Geometry check sheet. Reference: drawing and pictorial views, mm from the part's lowest x, y, z. A direction names the side the tool comes from. Give positions to 0.01 mm unless a question says otherwise; leave off trailing zeros. Order: outer loops, then holes, each group sorted by start corner. A loop starts at its lowest first (then second) coordinate and runs counter-clockwise, first axis right, second up.
Item 1: Release check for a two-part mould opening along X. For the marked faces 3, 4 and 5 record: released by +X, released by -X, zero draft, split by the parting line, or undercut.
Item 2: Sectioned sample at C-C on x = 32.5. Record the boundary of the cut face in (y, z).
Item 3: Gauge pin test, flat ends, axial feed: P1, Ø1, axis at x = 28, z = 1, coming from the -Y side; P2, Ø10, axis at x = 25.5, y = 30.5, coming from the -Z side; P3, Ø0.9, axis at y = 44.5, z = 1.5, coming from the -X side; P4, Ø1.2, axis at y = 38, z = 2.5, coming from the -X side. Record the tip position at first contact, or that the pin passes through.
Item 4: Access from +Z, -Z, +X, -X, +Y, -Y to the whole of each face (thin tool, end or side, straight path). Record for the marked faces 1 and 2.
Item 5: Sectioned sample at B-B on y = 19. Record the boundary of the cut face in (x, z).
Item 6: Sectioned sample at D-D on z = 0.5. Record the boundary of the cut face in (x, y).
Item 7: Material ranges on line 1 along Y through (x, z) = (18.25, 1.3); line 2 along Y through (x, z) = (18.25, 1.75); line 3 along Y through (x, z) = (25, 0.35), recorded low to high.
Item 8: Sectioned sample at A-A on x = 18.25. Record the boundary of the cut face in (y, z), and give its area (3 significant figures).
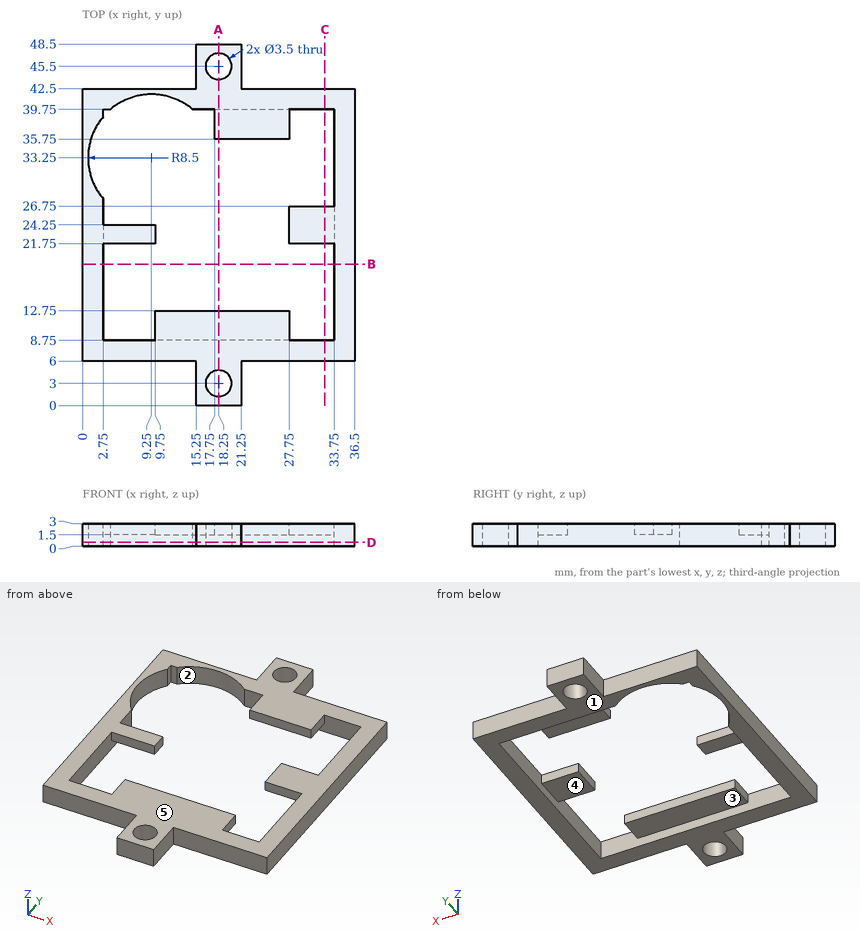
Report:
1. face 3: undercut
1. face 4: undercut
1. face 5: zero draft
2. outline: (6, 0) - (8.75, 0) - (8.75, 3) - (6, 3) - close; (21.75, 1.5) - (26.75, 1.5) - (26.75, 3) - (21.75, 3) - close; (39.75, 0) - (42.5, 0) - (42.5, 3) - (39.75, 3) - close
3. P1: stops at y = 6
3. P2: stops at z = 1.5
3. P3: stops at x = 15.25
3. P4: stops at x = 0
4. face 1: -Z, +X, -X, +Y, -Y
4. face 2: +Z, -Z
5. outline: (0, 0) - (2.75, 0) - (2.75, 3) - (0, 3) - close; (33.75, 0) - (36.5, 0) - (36.5, 3) - (33.75, 3) - close
6. outline: (0, 6) - (15.25, 6) - (15.25, 0) - (21.25, 0) - (21.25, 6) - (36.5, 6) - (36.5, 42.5) - (21.25, 42.5) - (21.25, 48.5) - (15.25, 48.5) - (15.25, 42.5) - (0, 42.5) - close; hole (2.75, 8.75) - (33.75, 8.75) - (33.75, 39.75) - (14.73, 39.75) arc R8.5 ccw to (3.77, 39.75) - (2.75, 39.75) - (2.75, 38.73) arc R8.5 ccw to (2.75, 27.77) - close; hole circle Ø3.5 at (18.25, 3); hole circle Ø3.5 at (18.25, 45.5)
7. line 1: y = 0 to 1.25, 4.75 to 8.75, 39.75 to 43.75, 47.25 to 48.5
7. line 2: y = 0 to 1.25, 4.75 to 12.75, 35.75 to 43.75, 47.25 to 48.5
7. line 3: y = 6 to 8.75, 39.75 to 42.5
8. outline: (0, 0) - (1.25, 0) - (1.25, 3) - (0, 3) - close; (4.75, 0) - (8.75, 0) - (8.75, 1.5) - (12.75, 1.5) - (12.75, 3) - (4.75, 3) - close; (35.75, 1.5) - (39.75, 1.5) - (39.75, 0) - (43.75, 0) - (43.75, 3) - (35.75, 3) - close; (47.25, 0) - (48.5, 0) - (48.5, 3) - (47.25, 3) - close
8. area: 43.5 mm2
